The model under review builds one solid part; all positions refer to its coordinate system, in mm. Round coordinates to 2 decimals unless told otherwise and drop trailing zeros. Order: outer loops, then holes, each group sorted by start corner. A loop starts at its lowest first (then second) coordinate and runs counter-clockwise, first axis right, second up.
from build123d import *

# Parameters (mm, degrees)
F_4_40_TAPPED_HOLE1_D           = 2.2606
F_4_40_TAPPED_HOLE1_DEPTH       = 10.414
F_4_40_TAPPED_HOLE1_CSINK_D     = 3.175
F_4_40_TAPPED_HOLE1_CSINK_ANGLE = 60
F_4_40_TAPPED_HOLE1_TIP         = 0.679152758


with BuildPart() as part:
    # Sketch3 → Revolve1 (revolve)
    with BuildSketch(Plane.XY, mode=Mode.PRIVATE) as revolve1_sk:
        Polygon((0, 0), (0, -1.9685), (2.921, -1.9685), (2.921, -2.3876), (21.844, -2.3876), (21.844, 0), align=None)
    revolve(revolve1_sk.sketch.rotate(Axis((0, 0, 0), (1, 0, 0)), 270), axis=Axis((0, 0, 0), (1, 0, 0)))

    # #4-40 Tapped Hole1
    with Locations(Plane.ZY):
        with Locations((0, 0)):
            CounterSinkHole(F_4_40_TAPPED_HOLE1_D / 2, F_4_40_TAPPED_HOLE1_CSINK_D / 2, depth=F_4_40_TAPPED_HOLE1_DEPTH, counter_sink_angle=F_4_40_TAPPED_HOLE1_CSINK_ANGLE)
            with Locations((0, 0, -(F_4_40_TAPPED_HOLE1_DEPTH + F_4_40_TAPPED_HOLE1_TIP / 2))):  # 118° drill point
                Cone(0, F_4_40_TAPPED_HOLE1_D / 2, F_4_40_TAPPED_HOLE1_TIP, mode=Mode.SUBTRACT)


solid = part.part
(1) We need section A-A (x = 12). Give the boundary of the cut face in (y, z), and give its area (3 significant figures).
(2) The part is to be moulded in two halves that separate along Y. For faces 1 (the cylindrical face through (5.67, -1.103, 0.245)), 2 (the cylindrical face through (12.51, 2.33, -0.52)), 3 (the flat face through (21.844, 0, 0)), say which applies: pulls with the +Y half, pulls with the -Y half, needs draft (parallel to the pull), parting line crosses it, or undercut.
(3) Clearance check with flat-ended pins moving along their axes: P1, Ø1.5, axis at x = 17.5, z = -1.5, coming from the -Y side; P2, Ø1.4, axis at y = 0, z = 0, coming from the -X side; P3, Ø2, axis at x = 11, y = -1.5, coming from the -Z side. State where each tip first meets the part, or that it passes through.
(4) We need section B-B (x = 6.5). Give the boundary of the cut face in (y, z), and give its area (3 significant figures).
(5) To check wall thickness, follow L1, parallel to Y at x = 8.75, z = 0; L2, parallel to X at y = 0.65, z = 2; L3, parallel to Z at x = 14.25, y = 1.35. State the ranges of each line that lie inside material, in increasing order.
Verdict:
1. outline: circle Ø4.78 at (0, 0)
1. area: 17.9 mm2
2. face 1: undercut
2. face 2: parting line crosses it
2. face 3: needs draft
3. P1: stops at y = -2.27
3. P2: stops at x = 10.67
3. P3: stops at z = -2.33
4. outline: circle Ø4.78 at (0, 0); hole circle Ø2.26 at (0, 0)
4. area: 13.9 mm2
5. L1: y = -2.39 to -1.13, 1.13 to 2.39
5. L2: x = 2.92 to 21.84
5. L3: z = -1.97 to 1.97
